```python
from build123d import *

# Parameters (mm, degrees)
SKETCH3_W           = 30
SKETCH3_H           = 72.5
BOSS_EXTRUDE2_DEPTH = 15.95
SKETCH7_W           = 20.5
SKETCH7_H           = 41
CUT_EXTRUDE5_DEPTH  = 8
SKETCH8_W           = 30
SKETCH8_H           = 35
CUT_EXTRUDE6_DEPTH  = 9.95
CUT_EXTRUDE7_DEPTH  = 50.683649222
SKETCH10_R          = 3.1
CUT_EXTRUDE8_DEPTH  = 50.683649222
CUT_EXTRUDE9_REACH  = 44.349
SKETCH11_R          = 1.6
CUT_EXTRUDE10_REACH = 42.996
SKETCH12_R          = 1.6
SKETCH13_W          = 7
SKETCH13_H          = 7
SKETCH13_R          = 1.6
BOSS_EXTRUDE3_DEPTH = 4


with BuildPart() as part:
    # Sketch3 → Boss-Extrude2 (new body)
    with BuildSketch(Plane(origin=(0, 0, 0), x_dir=(1, 0, 0), z_dir=(0, 1, 0))):
        Rectangle(SKETCH3_W, SKETCH3_H)
    extrude(amount=BOSS_EXTRUDE2_DEPTH)

    # Sketch7 → Cut-Extrude5 (cut)
    with BuildSketch(Plane.XZ):
        with Locations((0.25, 9)):
            Rectangle(SKETCH7_W, SKETCH7_H)
    extrude(amount=-CUT_EXTRUDE5_DEPTH, mode=Mode.SUBTRACT)

    # Sketch8 → Cut-Extrude6 (cut)
    with BuildSketch(Plane(origin=(0, 15.95, 0), x_dir=(1, 0, 0), z_dir=(0, 1, 0))):
        with Locations((0, 1.25)):
            Rectangle(SKETCH8_W, SKETCH8_H)
    extrude(amount=-CUT_EXTRUDE6_DEPTH, mode=Mode.SUBTRACT)

    # Sketch9 → Cut-Extrude7 (cut, through all)
    with BuildSketch(Plane(origin=(15, 0, 0), x_dir=(0, 0, -1), z_dir=(1, 0, 0))):
        Polygon((-36.25, 15.95), (-33.75, 15.95), (-33.75, 9.05), (-27.25, 9.05), (-27.25, 4.05), (-36.25, 4.05), align=None)
    extrude(amount=-CUT_EXTRUDE7_DEPTH, mode=Mode.SUBTRACT)

    # Sketch10 → Cut-Extrude8 (cut, through all)
    with BuildSketch(Plane(origin=(15, 0, 0), x_dir=(0, 0, -1), z_dir=(1, 0, 0))):
        with Locations((24.25, 16)):
            Circle(SKETCH10_R)
        with Locations((-21.75, 16)):
            Circle(SKETCH10_R)
    extrude(amount=-CUT_EXTRUDE8_DEPTH, mode=Mode.SUBTRACT)

    # Sketch11 → Cut-Extrude9 (cut, up to next)
    with BuildSketch(Plane(origin=(0, 15.95, 0), x_dir=(1, 0, 0), z_dir=(0, 1, 0)), mode=Mode.PRIVATE) as cut_extrude9_sk1:
        with Locations(Location((-9.5, -30.25, 0), (0, 0, 270))):
            Circle(SKETCH11_R)
    cut_extrude9_tool1 = extrude(cut_extrude9_sk1.sketch, amount=-CUT_EXTRUDE9_REACH, mode=Mode.PRIVATE) & part.part
    # Sketch11 → Cut-Extrude9 (cut, up to next)
    with BuildSketch(Plane(origin=(0, 15.95, 0), x_dir=(1, 0, 0), z_dir=(0, 1, 0)), mode=Mode.PRIVATE) as cut_extrude9_sk2:
        with Locations(Location((9.5, -30.25, 0), (0, 0, 270))):
            Circle(SKETCH11_R)
    cut_extrude9_tool2 = extrude(cut_extrude9_sk2.sketch, amount=-CUT_EXTRUDE9_REACH, mode=Mode.PRIVATE) & part.part
    # Sketch11 → Cut-Extrude9 (cut, up to next)
    with BuildSketch(Plane(origin=(0, 15.95, 0), x_dir=(1, 0, 0), z_dir=(0, 1, 0)), mode=Mode.PRIVATE) as cut_extrude9_sk3:
        with Locations(Location((-9.5, 30, 0), (0, 0, 270))):
            Circle(SKETCH11_R)
    cut_extrude9_tool3 = extrude(cut_extrude9_sk3.sketch, amount=-CUT_EXTRUDE9_REACH, mode=Mode.PRIVATE) & part.part
    # Sketch11 → Cut-Extrude9 (cut, up to next)
    with BuildSketch(Plane(origin=(0, 15.95, 0), x_dir=(1, 0, 0), z_dir=(0, 1, 0)), mode=Mode.PRIVATE) as cut_extrude9_sk4:
        with Locations(Location((9.5, 30, 0), (0, 0, 270))):
            Circle(SKETCH11_R)
    cut_extrude9_tool4 = extrude(cut_extrude9_sk4.sketch, amount=-CUT_EXTRUDE9_REACH, mode=Mode.PRIVATE) & part.part
    add(cut_extrude9_tool1.solids().sort_by_distance((-9.5, 15.95, 30.25))[0], mode=Mode.SUBTRACT)
    add(cut_extrude9_tool2.solids().sort_by_distance((9.5, 15.95, 30.25))[0], mode=Mode.SUBTRACT)
    add(cut_extrude9_tool3.solids().sort_by_distance((-9.5, 15.95, -30))[0], mode=Mode.SUBTRACT)
    add(cut_extrude9_tool4.solids().sort_by_distance((9.5, 15.95, -30))[0], mode=Mode.SUBTRACT)

    # Sketch12 → Cut-Extrude10 (cut, up to next)
    with BuildSketch(Plane(origin=(0, 4.05, 0), x_dir=(1, 0, 0), z_dir=(0, 1, 0)), mode=Mode.PRIVATE) as cut_extrude10_sk1:
        with Locations(Location((-5, -33, 0), (0, 0, 270))):
            Circle(SKETCH12_R)
    cut_extrude10_tool1 = extrude(cut_extrude10_sk1.sketch, amount=-CUT_EXTRUDE10_REACH, mode=Mode.PRIVATE) & part.part
    # Sketch12 → Cut-Extrude10 (cut, up to next)
    with BuildSketch(Plane(origin=(0, 4.05, 0), x_dir=(1, 0, 0), z_dir=(0, 1, 0)), mode=Mode.PRIVATE) as cut_extrude10_sk2:
        with Locations(Location((5, -33, 0), (0, 0, 270))):
            Circle(SKETCH12_R)
    cut_extrude10_tool2 = extrude(cut_extrude10_sk2.sketch, amount=-CUT_EXTRUDE10_REACH, mode=Mode.PRIVATE) & part.part
    # Sketch12 → Cut-Extrude10 (cut, up to next)
    with BuildSketch(Plane(origin=(0, 4.05, 0), x_dir=(1, 0, 0), z_dir=(0, 1, 0)), mode=Mode.PRIVATE) as cut_extrude10_sk3:
        with Locations(Location((-5, 15, 0), (0, 0, 270))):
            Circle(SKETCH12_R)
    cut_extrude10_tool3 = extrude(cut_extrude10_sk3.sketch, amount=-CUT_EXTRUDE10_REACH, mode=Mode.PRIVATE) & part.part
    # Sketch12 → Cut-Extrude10 (cut, up to next)
    with BuildSketch(Plane(origin=(0, 4.05, 0), x_dir=(1, 0, 0), z_dir=(0, 1, 0)), mode=Mode.PRIVATE) as cut_extrude10_sk4:
        with Locations(Location((5, 15, 0), (0, 0, 270))):
            Circle(SKETCH12_R)
    cut_extrude10_tool4 = extrude(cut_extrude10_sk4.sketch, amount=-CUT_EXTRUDE10_REACH, mode=Mode.PRIVATE) & part.part
    add(cut_extrude10_tool1.solids().sort_by_distance((-5, 4.05, 33))[0], mode=Mode.SUBTRACT)
    add(cut_extrude10_tool2.solids().sort_by_distance((5, 4.05, 33))[0], mode=Mode.SUBTRACT)
    add(cut_extrude10_tool3.solids().sort_by_distance((-5, 4.05, -15))[0], mode=Mode.SUBTRACT)
    add(cut_extrude10_tool4.solids().sort_by_distance((5, 4.05, -15))[0], mode=Mode.SUBTRACT)

    # Sketch13 → Boss-Extrude3 (add)
    # profile 1 of 2: a face of its own
    with BuildSketch(Plane(origin=(0, 0, -36.25), x_dir=(-1, 0, 0), z_dir=(0, 0, -1))):
        with Locations((18.5, 12.45)):
            Rectangle(SKETCH13_W, SKETCH13_H)
        with Locations((18.5, 12.45)):
            Circle(SKETCH13_R, mode=Mode.SUBTRACT)
    # profile 2 of 2: a face of its own
    with BuildSketch(Plane(origin=(0, 0, -36.25), x_dir=(-1, 0, 0), z_dir=(0, 0, -1))):
        with Locations((-18.5, 12.45)):
            Rectangle(SKETCH13_W, SKETCH13_H)
        with Locations((-18.5, 12.45)):
            Circle(SKETCH13_R, mode=Mode.SUBTRACT)
    extrude(amount=-BOSS_EXTRUDE3_DEPTH)


solid = part.part
```
Geometry check sheet. Reference: the model listing, model coordinates, mm. A direction names the side the tool comes from. Coordinates: 2 decimals unless noted, no trailing zeros. Order: outer loops, then holes, each group sorted by start corner. A loop starts at its lowest first (then second) coordinate and runs counter-clockwise, first axis right, second up.
Item 1: Section check A-A (z = 33). Enter the section's corners in (x, y), plus the area to 3 significant figures.
Item 2: Tool access check on faces 4 (the flat face through (0, 9.05, 31)), 5 (the cylindrical face through (8.5, 12.5, 29)), 6 (the flat face through (0, 8, 22)), 7 (the flat face through (19, 8.95, -34)). Record the directions out of +Z, -Z, +X, -X, +Y, -Y that give a thin tool (end or side, any length) a straight path to the whole face; none if there is none.
Item 3: Section check B-B (x = 5). Enter the section's corners in (y, z).
Item 4: Depth check by flat-ended pin: pin 1 (2 mm diameter, centred on x = 1, y = 11, fed in from +Z); pin 2 (12 mm diameter, centred on x = -1, z = 20, fed in from -Y); pin 3 (3 mm diameter, centred on x = -5, z = -16.5, fed in from +Y). Enter the tip coordinate at first touch or a pass-through.
Item 5: Scan lines: line 1 along X through (y, z) = (11.75, 30.25); line 2 along X through (y, z) = (1.1, -15); line 3 along X through (y, z) = (4.75, -7.5). Record each from-to range of solid material in increasing order.
Item 6: Section check C-C (x = -18.5). Enter the section's corners in (y, z).
Item 7: Mould release check, pull along Y, two halves, no side actions. Record for faces 1 (the cylindrical face through (-18.15, 10.89, -34.28)), 2 (the flat face through (-5, 4.05, -15)), 3 (the flat face through (-15, 4, 1)): released by +Y, released by -Y, zero draft, split by the parting line, or undercut.
Item 8: Section check D-D (z = -30). Enter the section's corners in (x, y), plus the area to 3 significant figures.
Check sheet entries:
1. outline: (-15, 0) - (-6.6, 0) - (-6.6, 4.05) - (-15, 4.05) - close; (-15, 9.05) - (15, 9.05) - (15, 15.95) - (-15, 15.95) - close; (-3.4, 0) - (3.4, 0) - (3.4, 4.05) - (-3.4, 4.05) - close; (6.6, 0) - (15, 0) - (15, 4.05) - (6.6, 4.05) - close
1. area: 303 mm2
2. face 4: +Z, +X, -X
2. face 5: +Y
2. face 6: +Z, -Y
2. face 7: +Z, -Z, +X, -Y
3. outline: (0, -36.25) - (15.95, -36.25) - (15.95, -27.35) arc R3.1 cw to (15.95, -21.15) - (15.95, -18.75) - (6, -18.75) - (6, -11.5) - (0, -11.5) - (0, -13.4) - (4.05, -13.4) - (4.05, -16.6) - (0, -16.6) - close; (0, 29.5) - (4.05, 29.5) - (4.05, 31.4) - (0, 31.4) - close; (0, 34.6) - (4.05, 34.6) - (4.05, 36.25) - (0, 36.25) - close; (8, 16.25) - (15.95, 16.25) - (15.95, 18.65) arc R3.1 cw to (15.95, 24.85) - (15.95, 33.75) - (9.05, 33.75) - (9.05, 27.25) - (8, 27.25) - close
4. pin 1: stops at z = 33.75
4. pin 2: stops at y = 8
4. pin 3: stops at y = 6
5. line 1: x = -15 to -11.1, -7.9 to 7.9, 11.1 to 15
5. line 2: x = -15 to -6.6, -3.4 to 3.4, 6.6 to 15
5. line 3: x = -15 to -10, 10.5 to 15
6. outline: (8.95, -36.25) - (10.85, -36.25) - (10.85, -32.25) - (8.95, -32.25) - close; (14.05, -36.25) - (15.95, -36.25) - (15.95, -32.25) - (14.05, -32.25) - close
7. face 1: undercut
7. face 2: released by -Y
7. face 3: zero draft
8. outline: (-15, 0) - (-11.1, 0) - (-11.1, 15.95) - (-15, 15.95) - close; (-7.9, 0) - (7.9, 0) - (7.9, 15.95) - (-7.9, 15.95) - close; (11.1, 0) - (15, 0) - (15, 15.95) - (11.1, 15.95) - close
8. area: 376 mm2
